Can you work these out from the model? Positions are in its coordinate system, mm. A direction names the side the tool comes from. Coordinates: 2 decimals unless noted, no trailing zeros. Write each loop counter-clockwise with the first axis right and the second up, starting at its lowest first coordinate (ties: lowest second). Pieces come first, ordered by that corner, then holes. Notation, with made-up numbers: (20, 1.5) - (39, 1.5) arc R21 ccw to (39, 28.5) - close; hole circle Ø1 at (67, 84). An arc over 180 degrees is marked (long way). Use one line per item in the form item = value. Start each with the question number.
(1) If we section it at C-C on z = 13.5: Please give me the cut outline in (x, y), then the cut area to 3 significant figures.
(2) If we section it at B-B on y = -17.5: Please give me the cut outline in (x, z), then the cut area to 3 significant figures.
(3) If I drill on probe 1 along Z at (x, y) = (4, -28.5); probe 2 along Z at (x, y) = (8.25, -12); probe 3 along Y at (x, z) = (22.75, 27), over which ranges is the centre line in solid material (lowest first)? Write a range as from..to.
(4) If we section it at A-A on x = 6.5: Please give me the cut outline in (y, z) (3 decimals).
(5) On a 3-axis mill with a long thin cutter (end or side, diameter ignored), from which of +Z, -Z, +X, -X, +Y, -Y can I reach the whole of each face in a straight line? I mean faces 1 (the face through (14, -27.026, 17)), 2 (the face through (2.914, -28.566, 20.024)). Say none if no direction works.
(6) Thinking about a two-plate mould opening in Y: for faces 3 (the face through (2.91, -28.57, 6.41)), 4 (the face through (14, -30.15, 15)), 5 (the face through (11.51, -9.26, 1.58)), which applies, pulls with the +Y half, pulls with the -Y half, needs draft (parallel to the pull), parting line crosses it, or undercut?
(7) For pin 1 Ø3 at (x, y) = (19.5, -12) entering from +Z; pin 2 Ø3 at (x, y) = (16, -26) entering from +Z; pin 3 Ø12.5 at (x, z) = (11.5, 18) entering from +Y, each with a flat end and sliding along its axis, tell me the tip position at first contact or that it passes through.
```python
from build123d import *

# Parameters (mm, degrees)
BOSS_EXTRUDE1_DEPTH     = 28.2702
SKETCH2_R               = 3.556
SKETCH2_R_2             = 1.524
SKETCH2_R_3             = 2.032
MOTOR_MOUNT_HOLES_DEPTH = 50.437835996
SKETCH3_R               = 1.7018
PLATE_MOUNT_HOLES_DEPTH = 50.444256141
FILLET1_R               = 1.651
FILLET2_R               = 0.889
FILLET3_R               = 0.635


with BuildPart() as part:
    # Sketch1 → Boss-Extrude1 (new body)
    with BuildSketch(Plane(origin=(0, 0, 0), x_dir=(0, 0, -1), z_dir=(1, 0, 0))):
        Polygon((0, 0), (0, -30.1498), (-30.2514, -30.1498), (-30.2514, -27.0256), (-3.1242, -27.0256), (-3.1242, 0), align=None)
    extrude(amount=BOSS_EXTRUDE1_DEPTH)

    # Sketch2 → Motor_Mount_holes (cut, through all)
    with BuildSketch(Plane.XY.offset(3.1242)):
        with Locations((14.1351, -11.6586)):
            Circle(SKETCH2_R)
        with Locations((14.1351, -3.1496)):
            Circle(SKETCH2_R_2)
        with Locations((5.4356, -11.6586)):
            Circle(SKETCH2_R_3)
        with Locations(Location((22.8346, -11.6586, 0), (0, 0, 180))):
            Circle(SKETCH2_R_3)
        with Locations(Location((14.1351, -20.1676, 0), (0, 0, 180))):
            Circle(SKETCH2_R_2)
    extrude(amount=-MOTOR_MOUNT_HOLES_DEPTH, mode=Mode.SUBTRACT)

    # Sketch3 → Plate_Mount_Holes (cut, through all)
    with BuildSketch(Plane(origin=(0, -27.0256, 0), x_dir=(1, 0, 0), z_dir=(0, 1, 0))):
        with Locations(Location((24.3205, -7.7597, 0), (0, 0, 270))):
            Circle(SKETCH3_R)
        with Locations(Location((3.9497, -7.7597, 0), (0, 0, 270))):
            Circle(SKETCH3_R)
        with Locations(Location((3.9497, -21.3741, 0), (0, 0, 270))):
            Circle(SKETCH3_R)
        with Locations(Location((24.3205, -21.3741, 0), (0, 0, 270))):
            Circle(SKETCH3_R)
    extrude(amount=-PLATE_MOUNT_HOLES_DEPTH, mode=Mode.SUBTRACT)

    # Fillet1
    fillet1_edges = [part.edges().sort_by_distance(p)[0] for p in [
        (14.1351, -27.0256, 3.1242),
    ]]
    fillet(fillet1_edges, radius=FILLET1_R)

    # Fillet2
    fillet2_edges = [part.edges().sort_by_distance(p)[0] for p in [
        (14.1351, -30.1498, 0),
    ]]
    fillet(fillet2_edges, radius=FILLET2_R)

    # Fillet3
    fillet3_edges = [part.edges().sort_by_distance(p)[0] for p in [
        (14.1351, 0, 0),
        (14.1351, -30.1498, 30.2514),
        (14.1351, -27.0256, 30.2514),
        (14.1351, 0, 3.1242),
    ]]
    fillet(fillet3_edges, radius=FILLET3_R)


solid = part.part
```
Reported:
q1.outline = (0, -30.15) - (28.27, -30.15) - (28.27, -27.03) - (0, -27.03) - close
q1.area = 88.3 mm2
q2.outline = (0, 0) - (28.27, 0) - (28.27, 3.12) - (0, 3.12) - close
q2.area = 88.3 mm2
q3.probe_1 = 0..6.06, 9.46..19.67, 23.08..30.25
q3.probe_2 = 0..3.12
q3.probe_3 = -30.15..-27.03
q4.outline = (-30.15, 0.889) arc R0.889 ccw to (-29.261, 0) - (-13.39, 0) - (-13.39, 3.124) - (-25.375, 3.124) arc R1.651 cw to (-27.026, 4.775) - (-27.026, 29.616) arc R0.635 ccw to (-27.661, 30.251) - (-29.515, 30.251) arc R0.635 ccw to (-30.15, 29.616) - close; (-9.928, 0) - (-0.635, 0) arc R0.635 ccw to (0, 0.635) - (0, 2.489) arc R0.635 ccw to (-0.635, 3.124) - (-9.928, 3.124) - close
q5.face_1 = +Z, +X, -X, +Y
q5.face_2 = +Y, -Y
q6.face_3 = needs draft
q6.face_4 = pulls with the -Y half
q6.face_5 = undercut
q7.pin_1 = 3.12
q7.pin_2 = 30.23
q7.pin_3 = -27.03
